Model file for the job. Use its own axes, mm. Face numbers are marked on the shaded views. A direction names the side the tool comes from. Round coordinates to 2 decimals unless told otherwise and drop trailing zeros. Loops run counter-clockwise (first coordinate to the right, second up) from the corner with the lowest first, then second, coordinate; pieces in that order, holes last. Notation, with made-up numbers: M -8.5,68.25 L 44.5,68.25 A14 cw 44.5,82.25 Z; hole C -14,72.5 d6. An arc over 180 degrees is marked long. Use a Markdown table: item, result. Add a question column.
Item 1: Saw through at A-A on y = 4.25. Write the cut outline in (x, z), then the cut area to 3 significant figures.
Item 2: Pin check, flat tips, straight feed: P1, Ø2, axis at x = 3, y = 4.25, coming from the +Z side; P2, Ø0.5, axis at y = 5.5, z = 1.5, coming from the -X side; P3, Ø0.6, axis at x = 11, z = 1, coming from the -Y side. Stop position of each tip, or through.
Item 3: Saw through at C-C on x = 3. Write the cut outline in (y, z).
Item 4: Two-plate mould, pull along X, no slides. Class the marked faces 1, 2 and 3: +X half, -X half, draft (parallel to the pull), parting line (faces both ways), or undercut.
Item 5: Saw through at D-D on x = 11.75. Write the cut outline in (y, z).
Item 6: Wall check: L1, parallel to X at y = 4.5, z = 1.4; L2, parallel to X at y = 4.85, z = 1.65; L3, parallel to Y at x = 12.25, z = 1.5. Give the ranges that are in metal, low to high. Write a range as from..to.
Item 7: Tool access for the marked faces 4 and 5: list every direction of +Z, -Z, +X, -X, +Y, -Y with a clear straight run to the whole face (end or side of a thin tool).
Item 8: Saw through at B-B on z = 1.7. Write the cut outline in (x, y).
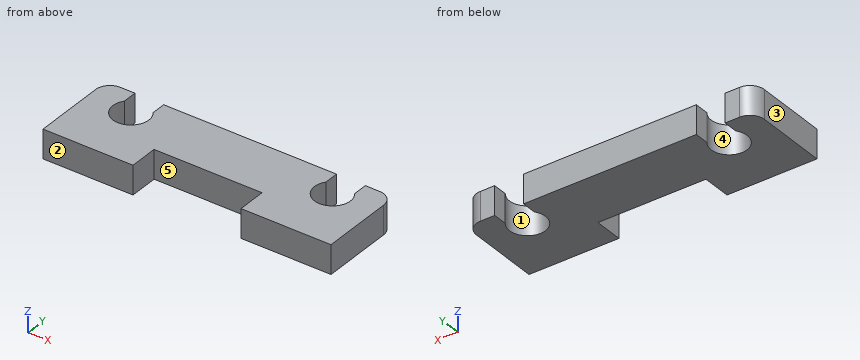
```python
from build123d import *

# Parameters (mm, degrees)
BOSS_EXTRUDE1_DEPTH = 2


with BuildPart() as part:
    # Model → Boss-Extrude1 (new body)
    with BuildSketch(Plane.XY):
        with BuildLine():
            Line((6.25, 2), (13.75, 2))
            Line((13.75, 2), (13.75, 0))
            Line((13.75, 0), (20, 0))
            Line((20, 0), (20, 5))
            ThreePointArc((20, 5), (19.707106781, 5.707106781), (19, 6))
            Line((19, 6), (18, 6))
            Line((18, 6), (18, 5))
            ThreePointArc((18, 5), (17, 3), (16, 5))
            Line((16, 5), (16, 6))
            Line((16, 6), (4, 6))
            Line((4, 6), (4, 5))
            ThreePointArc((4, 5), (3, 3), (2, 5))
            Line((2, 5), (2, 6))
            Line((2, 6), (1, 6))
            ThreePointArc((1, 6), (0.292893219, 5.707106781), (0, 5))
            Line((0, 5), (0, 0))
            Line((0, 0), (6.25, 0))
            Line((6.25, 0), (6.25, 2))
        make_face()
    extrude(amount=BOSS_EXTRUDE1_DEPTH)


solid = part.part
```
Entries:
| question | item | result |
|---|---|---|
| 1 | outline | M 0,0 L 1.75,0 L 1.75,2 L 0,2 Z; M 4.25,0 L 15.75,0 L 15.75,2 L 4.25,2 Z; M 18.25,0 L 20,0 L 20,2 L 18.25,2 Z |
| 1 | area | 30.0 mm2 |
| 2 | P1 | through |
| 2 | P2 | x = 0.03 |
| 2 | P3 | y = 2 |
| 3 | outline | M 0,0 L 3,0 L 3,2 L 0,2 Z |
| 4 | face 1 | undercut |
| 4 | face 2 | draft |
| 4 | face 3 | -X half |
| 5 | outline | M 2,0 L 6,0 L 6,2 L 2,2 Z |
| 6 | L1 | 0..1.78, 4.22..15.78, 18.22..20 |
| 6 | L2 | 0..1.9, 4.1..15.9, 18.1..20 |
| 6 | L3 | 2..6 |
| 7 | face 4 | +Z, -Z |
| 7 | face 5 | +Z, -Z, -Y |
| 8 | outline | M 0,0 L 6.25,0 L 6.25,2 L 13.75,2 L 13.75,0 L 20,0 L 20,5 A1 ccw 19,6 L 18,6 L 18,5 A1.25 cw long 16,5 L 16,6 L 4,6 L 4,5 A1.25 cw long 2,5 L 2,6 L 1,6 A1 ccw 0,5 Z |
